```python
from build123d import *

# Parameters (mm, degrees)
F4_DEPTH  = 8.9
F6_W      = 6
F6_H      = 10
F7_DEPTH  = 3.7
F8_R      = 0.3
F9_DEPTH  = 3.701
F11_DEPTH = 3


with BuildPart() as f4:
    # F3 (on Right) → F4 (new body)
    with BuildSketch(Plane.YZ):
        Polygon((0, 1.55), (0, 0), (0, -1.55), (19, -1.55), (19, 0), (19, 1.55), align=None)
    extrude(amount=F4_DEPTH)

    # F6 (on offset) → F7 (join)
    with BuildSketch(Plane.XY.offset(1.85)):
        with Locations((4.45, 12)):
            Rectangle(F6_W, F6_H)
    extrude(amount=-F7_DEPTH)

    # F8 (on offset) → F9 (cut, through all)
    with BuildSketch(Plane.XY.offset(1.85)):
        with BuildLine():
            ThreePointArc((1.4, 4), (1.6928932188, 3.2928932188), (2.4, 3))
            Line((2.4, 3), (6.5, 3))
            ThreePointArc((6.5, 3), (7.2071067812, 3.2928932188), (7.5, 4))
            Line((7.5, 4), (7.5, 5.5))
            ThreePointArc((7.5, 5.5), (7.2071067812, 6.2071067812), (6.5, 6.5))
            Line((6.5, 6.5), (2.4, 6.5))
            ThreePointArc((2.4, 6.5), (1.6928932188, 6.2071067812), (1.4, 5.5))
            Line((1.4, 5.5), (1.4, 4))
        make_face()
        with Locations((2.75, 15.64)):
            Circle(F8_R)
        with Locations((6.15, 15.64)):
            Circle(F8_R)
    extrude(amount=-F9_DEPTH, mode=Mode.SUBTRACT)

    # F10 (on face) → F11 (cut, through all)
    with BuildSketch(Plane.XZ):
        with BuildLine():
            Line((5.3, 1.55), (3.6, 1.55))
            Line((3.6, 1.55), (3.6, 0.6982120022))
            ThreePointArc((3.6, 0.6982120022), (4.45, -1.1), (5.3, 0.6982120022))
            Line((5.3, 0.6982120022), (5.3, 1.55))
        make_face()
    extrude(amount=-F11_DEPTH, mode=Mode.SUBTRACT)


solid = f4.part
```
Check sheet for the modelled part. Datum: model origin and axes. Units: mm. A direction names the side the tool comes from. Coordinates: 2 decimals unless noted, no trailing zeros. Loops run counter-clockwise (first coordinate to the right, second up) from the corner with the lowest first, then second, coordinate; pieces in that order, holes last.
1) Release check for a two-part mould opening along Y. For faces 1 (the face through (1.685, 3.301, 0.022)), 2 (the face through (1.4, 5, 0)), 3 (the face through (4, 19, 0)), 4 (the face through (4, 12, 1.85)) record: released by +Y, released by -Y, zero draft, split by the parting line, or undercut.
2) Sectioned sample at A-A (x = 4.45). Record the boundary of the cut face in (y, z), and give its area (3 significant figures).
3) Material ranges on probe 1 along Y at (x, z) = (3.5, 0.75); probe 2 along Y at (x, z) = (2.75, -1.1); probe 3 along Y at (x, z) = (3, 0.6), recorded low to high.
4) Sectioned sample at C-C (z = 0). Record the boundary of the cut face in (x, y), and give its area (3 significant figures).
5) Sectioned sample at D-D (y = 8.5). Record the boundary of the cut face in (x, z), and give its area (3 significant figures).
6) Access from +Z, -Z, +X, -X, +Y, -Y to the whole of each face (thin tool, end or side, straight path). Record for faces 5 (the face through (4.4, 1.5, -1.1)), 6 (the face through (5.3, 1, 1)), 7 (the face through (7.5, 5, 0)).
7) Sectioned sample at B-B (x = 2.75). Record the boundary of the cut face in (y, z).
Check sheet entries:
1. face 1: undercut
1. face 2: undercut
1. face 3: released by +Y
1. face 4: zero draft
2. outline: (0, -1.55) - (3, -1.55) - (3, -1.1) - (0, -1.1) - close; (6.5, -1.55) - (7, -1.55) - (7, -1.85) - (17, -1.85) - (17, -1.55) - (19, -1.55) - (19, 1.55) - (17, 1.55) - (17, 1.85) - (7, 1.85) - (7, 1.55) - (6.5, 1.55) - close
2. area: 46.1 mm2
3. probe 1: y = 0 to 3, 6.5 to 19
3. probe 2: y = 0 to 3, 6.5 to 15.34, 15.94 to 19
3. probe 3: y = 0 to 3, 6.5 to 15.47, 15.81 to 19
4. outline: (0, 0) - (3.35, 0) - (3.35, 3) - (2.4, 3) arc R1 cw to (1.4, 4) - (1.4, 5.5) arc R1 cw to (2.4, 6.5) - (6.5, 6.5) arc R1 cw to (7.5, 5.5) - (7.5, 4) arc R1 cw to (6.5, 3) - (5.55, 3) - (5.55, 0) - (8.9, 0) - (8.9, 19) - (0, 19) - close; hole circle Ø0.6 at (2.75, 15.64); hole circle Ø0.6 at (6.15, 15.64)
4. area: 141 mm2
5. outline: (0, -1.55) - (1.45, -1.55) - (1.45, -1.85) - (7.45, -1.85) - (7.45, -1.55) - (8.9, -1.55) - (8.9, 1.55) - (7.45, 1.55) - (7.45, 1.85) - (1.45, 1.85) - (1.45, 1.55) - (0, 1.55) - close
5. area: 31.2 mm2
6. face 5: -Y
6. face 6: +Z, -Y
6. face 7: +Z, -Z
7. outline: (0, -1.55) - (3, -1.55) - (3, 1.55) - (0, 1.55) - close; (6.5, -1.55) - (7, -1.55) - (7, -1.85) - (15.34, -1.85) - (15.34, 1.85) - (7, 1.85) - (7, 1.55) - (6.5, 1.55) - close; (15.94, -1.85) - (17, -1.85) - (17, -1.55) - (19, -1.55) - (19, 1.55) - (17, 1.55) - (17, 1.85) - (15.94, 1.85) - close
